Source: CAD feature listing. Evaluate the final solid. Frame: model axes, mm. Give positions to 0.01 mm unless a question says otherwise; leave off trailing zeros. Order: outer loops, then holes, each group sorted by start corner. A loop starts at its lowest first (then second) coordinate and runs counter-clockwise, first axis right, second up. Notation, with made-up numbers: M 47.25,40.25 L 52.25,40.25 A24 ccw 52.25,56.25 Z; hole C 1.5,78.25 d8. An arc over 180 degrees is marked long. Use CSV: the item, a comma, the result in double quotes. Start each with the question number.
Item 1: Section query A-A on z = 0. Return loops of the section in (x, y), and give its area (3 significant figures).
Item 2: First-contact query: pin 1 (10 mm diameter, centred on x = -108.5, y = 0, fed in from -Z); pin 2 (3 mm diameter, centred on y = -10.5, z = -4, fed in from -X); pin 3 (4 mm diameter, centred on x = -34.5, y = 2, fed in from -Z); pin 4 (0.8 mm diameter, centred on x = -19.5, y = 4.5, fed in from +Z). Flat tips, straight axial feed; report the tip coordinate or a pass-through.
Item 3: Ray query, probe 1 along Y at (x, z) = (-152, -10); probe 2 along Y at (x, z) = (-72.5, 4.75); probe 3 along Y at (x, z) = (71, 0). Return the intervals inside material, ascending. Write a range as from..to.
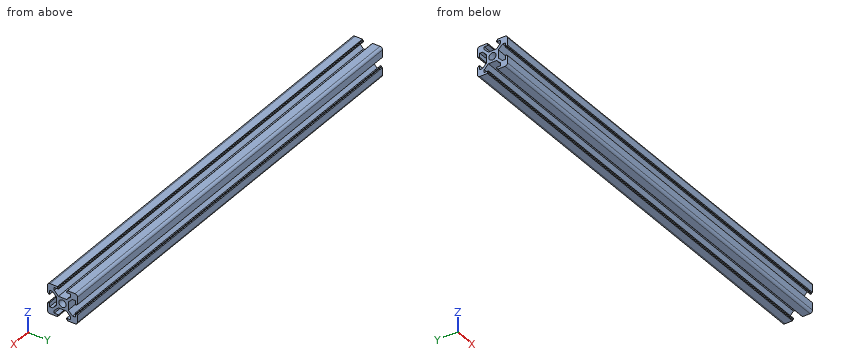
from build123d import *

# Parameters (mm, degrees)
SKETCH1_R                           = 3.65
BOSCHREXROTH_BOSCH_30X30_V2_1_DEPTH = 431.8


with BuildPart() as part:
    # Sketch1 → Boschrexroth BOSCH_30X30_V2(1) (new body)
    with BuildSketch(Plane(origin=(-215.9, 0, 0), x_dir=(0, 0, -1), z_dir=(1, 0, 0))):
        with BuildLine():
            Line((0, 5.8), (-4.03, 5.8))
            Line((-4.03, 5.8), (-8.25, 10.02))
            Line((-8.25, 10.02), (-8.25, 12.8))
            Line((-8.25, 12.8), (-4.1, 12.8))
            Line((-4.1, 12.8), (-4.1, 13.9))
            Line((-4.1, 13.9), (-5.1, 13.9))
            Line((-5.1, 13.9), (-5.1, 15))
            Line((-5.1, 15), (-12.5, 15))
            ThreePointArc((-12.5, 15), (-14.267766953, 14.267766953), (-15, 12.5))
            Line((-15, 12.5), (-15, 5.1))
            Line((-15, 5.1), (-13.9, 5.1))
            Line((-13.9, 5.1), (-13.9, 4.1))
            Line((-13.9, 4.1), (-12.8, 4.1))
            Line((-12.8, 4.1), (-12.8, 8.25))
            Line((-12.8, 8.25), (-10.02, 8.25))
            Line((-10.02, 8.25), (-5.8, 4.03))
            Line((-5.8, 4.03), (-5.8, 0))
            Line((-5.8, 0), (-5.8, -4.03))
            Line((-5.8, -4.03), (-10.02, -8.25))
            Line((-10.02, -8.25), (-12.8, -8.25))
            Line((-12.8, -8.25), (-12.8, -4.1))
            Line((-12.8, -4.1), (-13.9, -4.1))
            Line((-13.9, -4.1), (-13.9, -5.1))
            Line((-13.9, -5.1), (-15, -5.1))
            Line((-15, -5.1), (-15, -12.5))
            ThreePointArc((-15, -12.5), (-14.267766953, -14.267766953), (-12.5, -15))
            Line((-12.5, -15), (-5.1, -15))
            Line((-5.1, -15), (-5.1, -13.9))
            Line((-5.1, -13.9), (-4.1, -13.9))
            Line((-4.1, -13.9), (-4.1, -12.8))
            Line((-4.1, -12.8), (-8.25, -12.8))
            Line((-8.25, -12.8), (-8.25, -10.02))
            Line((-8.25, -10.02), (-4.03, -5.8))
            Line((-4.03, -5.8), (4.03, -5.8))
            Line((4.03, -5.8), (8.25, -10.02))
            Line((8.25, -10.02), (8.25, -12.8))
            Line((8.25, -12.8), (4.1, -12.8))
            Line((4.1, -12.8), (4.1, -13.9))
            Line((4.1, -13.9), (5.1, -13.9))
            Line((5.1, -13.9), (5.1, -15))
            Line((5.1, -15), (12.5, -15))
            ThreePointArc((12.5, -15), (14.267766953, -14.267766953), (15, -12.5))
            Line((15, -12.5), (15, -5.1))
            Line((15, -5.1), (13.9, -5.1))
            Line((13.9, -5.1), (13.9, -4.1))
            Line((13.9, -4.1), (12.8, -4.1))
            Line((12.8, -4.1), (12.8, -8.25))
            Line((12.8, -8.25), (10.02, -8.25))
            Line((10.02, -8.25), (5.8, -4.03))
            Line((5.8, -4.03), (5.8, 0))
            Line((5.8, 0), (5.8, 4.03))
            Line((5.8, 4.03), (10.02, 8.25))
            Line((10.02, 8.25), (12.8, 8.25))
            Line((12.8, 8.25), (12.8, 4.1))
            Line((12.8, 4.1), (13.9, 4.1))
            Line((13.9, 4.1), (13.9, 5.1))
            Line((13.9, 5.1), (15, 5.1))
            Line((15, 5.1), (15, 12.5))
            ThreePointArc((15, 12.5), (14.267766953, 14.267766953), (12.5, 15))
            Line((12.5, 15), (5.1, 15))
            Line((5.1, 15), (5.1, 13.9))
            Line((5.1, 13.9), (4.1, 13.9))
            Line((4.1, 13.9), (4.1, 12.8))
            Line((4.1, 12.8), (8.25, 12.8))
            Line((8.25, 12.8), (8.25, 10.02))
            Line((8.25, 10.02), (4.03, 5.8))
            Line((4.03, 5.8), (0, 5.8))
        make_face()
        Circle(SKETCH1_R, mode=Mode.SUBTRACT)
    extrude(amount=BOSCHREXROTH_BOSCH_30X30_V2_1_DEPTH)


solid = part.part
Verdict:
1,outline,"M -215.9,-5.8 L 215.9,-5.8 L 215.9,-3.65 L -215.9,-3.65 Z; M -215.9,3.65 L 215.9,3.65 L 215.9,5.8 L -215.9,5.8 Z"
1,area,"1,860 mm2"
2,pin 1,"z = -13.9"
2,pin 2,"through"
2,pin 3,"z = -5.8"
2,pin 4,"z = 13.9"
3,probe 1,"-15..-8.23, 8.23..15"
3,probe 2,"-13.9..-12.8, -6.52..6.52, 12.8..13.9"
3,probe 3,"-5.8..-3.65, 3.65..5.8"
